Could you check a few things on this model? Use its own coordinates, in mm. A direction names the side the tool comes from. Round coordinates to 2 decimals unless told otherwise and drop trailing zeros. Write each loop counter-clockwise with the first axis right and the second up, starting at its lowest first coordinate (ties: lowest second). Pieces come first, ordered by that corner, then holes. Notation, with made-up numbers: M 37.25,40 L 70.25,40 A6 cw 70.25,44 Z; hole C 17.5,10 d5. An arc over 180 degrees is marked long. One line per question, with ' | ' between items. Start each with the question number.
Solid Edge part; units mm, degrees
sketch "Sketch1" plane through (0, 0, 0) normal (0, 0, 1) x (1, 0, 0)
  line L0 (2, 0) -> (2, 16)
  line L1 (0, 16) -> (2, 16)
  line L2 (0, 0) -> (0, 16)
  line L3 (0, 0) -> (0, -4)
  line L4 (0, -4) -> (3.5, -4)
  line L5 (3.5, -4) -> (3.5, 0)
  line L6 (3.5, 0) -> (2, 0)
revolve "RevolvedProtrusion1" add sketch "Sketch1" angle 360 about axis through (0, 0, 0) along (0, 1, 0)
sketch "Sketch2" plane through (0, 0, 0) normal (1, 0, 0) x (0, 1, 0)
  line L0 (-4, 2.2215) -> (-2, 2.2215)
  line L1 (-0.7174, 0) -> (-2, 2.2215)
  line L2 (-4, 0) -> (-0.7174, 0)
  line L3 (-4, 0) -> (-4, 2.2215)
revolve "RevolvedCutout1" cut sketch "Sketch2" angle 360 about axis through (0, -4.5, 0) along (0, 1, 0)
sketch "Sketch3" plane through (0, -4, 0) normal (0, -1, 0) x (0, 0, 1)
  circle A0 centre (0, 0) radius 2.2215
  line L0 (-1.5, -0.866) -> (0, -1.7321)
  line L1 (0, -1.7321) -> (1.5, -0.866)
  line L2 (1.5, -0.866) -> (1.5, 0.866)
  line L3 (1.5, 0.866) -> (0, 1.7321)
  line L4 (0, 1.7321) -> (-1.5, 0.866)
  line L5 (-1.5, 0.866) -> (-1.5, -0.866)
extrude "Protrusion1" add sketch "Sketch3" against normal up to next
sketch "Sketch4" plane through (0, 0, 0) normal (0, 0, 1) x (1, 0, 0)
  line L0 (-1.7321, -4) -> (0, -4)
  line L1 (0, -4) -> (0, -3.5359)
  line L2 (0, -3.5359) -> (-1.7321, -4)
revolve "RevolvedCutout2" cut sketch "Sketch4" angle 360 about axis through (0, -4.5, 0) along (0, 1, 0)
fillet "Round1" radius 0.2 1 edges at (0, 0, -2)
fillet "Round2" radius 0.35 1 edges at (0, -4, -3.5)
chamfer "倒斜角_2" distance 0.2667 angle 45 1 edges at (0, 16, -2)
cosmetic_thread "螺纹_3" thread depth 12.8
properties part number "N2611-031H" material "铝 1060"
1. If we mould it in two halves opening along X, with no side actions, what happens to faces 4 (the face through (-2, 0, 2)), 5 (the face through (0, -3, 1.5)), 6 (the face through (-0.033, -0.78, 0.103)), 7 (the face through (3.233, -1.799, 1.341))? For each: released by +X, released by -X, zero draft, split by the parting line, or undercut.
2. I need wall thicknesses on line 1 along Y through (x, z) = (-2.75, 1.5); line 2 along Z through (x, y) = (0.75, -1.5); line 3 along Y through (x, z) = (1.5, -3). Which ranges of each line are inside material? Lowest first, please. Write a range as from..to.
3. Suppose I cut it at A-A (y = 15.25). Write out the boundary of the cut face in (x, z), and give its area (3 significant figures).
4. Which directions (+Z, -Z, +X, -X, +Y, -Y) give clear straight access to the entire face, cutting with the end or side of a thin tool? Please do faces 1 (the face through (0, 8, 2)), 2 (the face through (0, 16, 0)), 3 (the face through (-1.305, -2.809, -0.739)).
5. I'm going to push flat-ended pins straight in: P1, Ø0.5, axis at x = -0.5, y = -3, coming from the +Z side; P2, Ø3, axis at x = 2.5, y = 7.5, coming from the -Z side; P3, Ø1.5, axis at y = 6.5, z = 1, coming from the -X side. Where does each tip first touch, or does it pass through?
Computed:
1) face 4: zero draft | face 5: undercut | face 6: undercut | face 7: split by the parting line
2) line 1: y = -4..0 | line 2: z = -3.42..-1.13, 1.13..3.42 | line 3: y = -3.93..0
3) outline: C 0,0 d4 | area: 12.6 mm²
4) face 1: +Y | face 2: +Z, -Z, +X, -X, +Y | face 3: -Y
5) P1: stops at z = 3.49 | P2: stops at z = -1.73 | P3: stops at x = -1.98
